from build123d import *

# Parameters (mm, degrees)
PAD005_DEPTH        = 16
FILLET004_R         = 2.5
HOLE005_D           = 4.5
HOLE005_CBORE_D     = 5.6
HOLE005_CBORE_DEPTH = 4.4
SKETCH025_R         = 8.6
PAD007_DEPTH        = 8
PAD008_DEPTH        = 8


with BuildPart() as part:
    # Sketch021 → Pad005 (new body)
    with BuildSketch(Plane.XY):
        with BuildLine():
            Line((-4.795832, 11), (-21, 11))
            Line((-21, 11), (-21, 8))
            Line((-21, 8), (-4.123106, 8))
            ThreePointArc((-4.123106, -8), (9, 0), (-4.123106, 8))
            Line((-21, -8), (-4.123106, -8))
            Line((-21, -12), (-21, -8))
            Line((0, -12), (-21, -12))
            ThreePointArc((0, -12), (11.74734, 2.44949), (-4.795832, 11))
        make_face()
    extrude(amount=PAD005_DEPTH)

    # Fillet004
    fillet004_edges = [part.edges().sort_by_distance(p)[0] for p in [
        (-21, 9.5, 0),
        (-21, 9.5, 16),
        (-21, -10, 16),
        (-21, -10, 0),
    ]]
    fillet(fillet004_edges, radius=FILLET004_R)

    # Hole005 (through all)
    with Locations(Plane.XZ.offset(12)):
        with Locations((-13, 8)):
            CounterBoreHole(HOLE005_D / 2, HOLE005_CBORE_D / 2, HOLE005_CBORE_DEPTH)

    # Sketch025 → Pad007 (join)
    with BuildSketch(Plane.XY):
        with BuildLine():
            ThreePointArc((18.8, 19.2), (13.143146, 16.856854), (10.8, 11.2))
            Line((10.8, -11.2), (10.8, 11.2))
            ThreePointArc((10.8, -11.2), (13.143146, -16.856854), (18.8, -19.2))
            Line((55.2, -19.2), (18.8, -19.2))
            ThreePointArc((55.2, -19.2), (60.856854, -16.856854), (63.2, -11.2))
            Line((63.2, 11.2), (63.2, -11.2))
            ThreePointArc((63.2, 11.2), (60.856854, 16.856854), (55.2, 19.2))
            Line((18.8, 19.2), (55.2, 19.2))
        make_face()
        with Locations((37, 0)):
            Circle(SKETCH025_R, mode=Mode.SUBTRACT)
        with BuildLine():
            ThreePointArc((18.8, 18), (13.991674, 16.008326), (12, 11.2))
            Line((12, 11.2), (12, 1))
            Line((12, 1), (27.251154, 1))
            ThreePointArc((36.4, 9.781615), (30.213702, 7.070089), (27.251154, 1))
            Line((36.4, 18), (36.4, 9.781615))
            Line((18.8, 18), (36.4, 18))
        make_face(mode=Mode.SUBTRACT)
        with BuildLine():
            ThreePointArc((62, 11.2), (60.008326, 16.008326), (55.2, 18))
            Line((37.6, 18), (55.2, 18))
            Line((37.6, 9.781615), (37.6, 18))
            ThreePointArc((37.6, -9.781615), (46.8, 0), (37.6, 9.781615))
            Line((37.6, -18), (37.6, -9.781615))
            Line((55.2, -18), (37.6, -18))
            ThreePointArc((55.2, -18), (60.008326, -16.008326), (62, -11.2))
            Line((62, 11.2), (62, -11.2))
        make_face(mode=Mode.SUBTRACT)
        with BuildLine():
            ThreePointArc((12, -11.2), (13.991674, -16.008326), (18.8, -18))
            Line((36.4, -18), (18.8, -18))
            Line((36.4, -9.781615), (36.4, -18))
            ThreePointArc((27.251154, -1), (30.213702, -7.070089), (36.4, -9.781615))
            Line((12, -1), (27.251154, -1))
            Line((12, -11.2), (12, -1))
        make_face(mode=Mode.SUBTRACT)
    extrude(amount=PAD007_DEPTH)

    # Sketch026 → Pad008 (join)
    with BuildSketch(Plane.XY):
        with BuildLine():
            ThreePointArc((5.838182, 10.484066), (8.996246, 10.358804), (10.967642, 12.82916))
            Line((10.967642, 12.82916), (10.967642, -12.82916))
            ThreePointArc((10.967642, -12.82916), (8.996246, -10.358804), (5.838182, -10.484066))
            Line((5.838182, -10.484066), (4.427288, -7.950416))
            ThreePointArc((4.427288, -7.950416), (9.1, 0), (4.427288, 7.950416))
            Line((5.838182, 10.484066), (4.427288, 7.950416))
        make_face()
    extrude(amount=PAD008_DEPTH)


solid = part.part
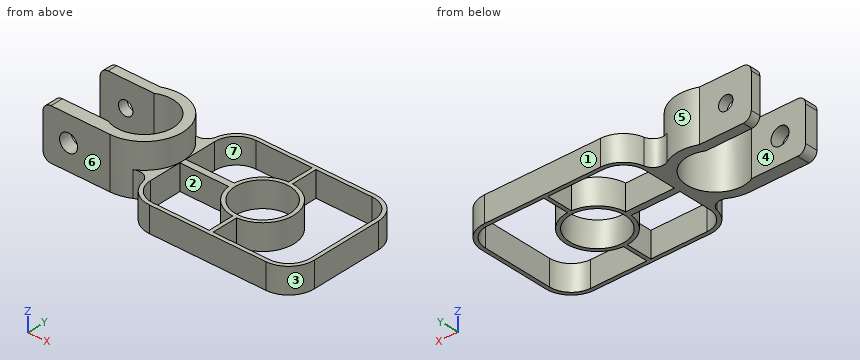
Part model, mm, in its own coordinate system. Face numbers are marked on the shaded views. A direction names the side the tool comes from. Coordinates: 2 decimals unless noted, no trailing zeros. Write each loop counter-clockwise with the first axis right and the second up, starting at its lowest first coordinate (ties: lowest second). Pieces come first, ordered by that corner, then holes. Notation, with made-up numbers: M 41.5,-12.5 L 93.5,-12.5 A18 ccw 93.5,15.5 Z; hole C -27,41.25 d7. An arc over 180 degrees is marked long. Return JSON: item names as keys, results as strings.
1. Saw through at C-C, the plane x = -13. Write the cut outline in (y, z), then the cut area to 3 significant figures.
Determined:
{"outline": "M -12,0 L -8,0 L -8,5.2 L -12,5.2 Z; M -12,10.8 L -8,10.8 L -8,16 L -12,16 Z; M 8,0 L 11,0 L 11,5.75 L 8,5.75 Z; M 8,10.25 L 11,10.25 L 11,16 L 8,16 Z", "area": "76.1 mm²"}
2. Saw through at B-B, the plane y = 0. Write the cut outline in (x, z).
Determined:
{"outline": "M 9,0 L 28.4,0 L 28.4,8 L 12,8 L 12,16 L 9,16 Z; M 45.6,0 L 46.8,0 L 46.8,8 L 45.6,8 Z; M 62,0 L 63.2,0 L 63.2,8 L 62,8 Z"}
3. Pull direction X, two halves, no side cores. Call the marked faces 1, 2 and 3: pulls with the +X half, pulls with the -X half, needs draft (parallel to the pull), parting line crosses it, or undercut.
Determined:
{"face 1": "needs draft", "face 2": "undercut", "face 3": "pulls with the +X half"}
4. Saw through at D-D, the plane z = 14.75. Write the cut outline in (x, y), then the cut area to 3 significant figures.
Determined:
{"outline": "M -20.67,-12 L 0,-12 A12 ccw long -4.8,11 L -20.67,11 L -20.67,8 L -4.12,8 A9 cw long -4.12,-8 L -20.67,-8 Z", "area": "241 mm²"}
5. Probe L1, parallel to Y at x = 18.5, z = 3.75; L2, parallel to Z at x = -13, y = -9; L3, parallel to Y at x = 51, z = 3.5. List the from-to ranges inside material, lowest first.
Determined:
{"L1": "-19.19 to -17.99, -1 to 1, 17.99 to 19.19", "L2": "0 to 5.2, 10.8 to 16", "L3": "-19.2 to -18, 18 to 19.2"}
6. Saw through at A-A, the plane x = 23. Write the cut outline in (y, z).
Determined:
{"outline": "M -19.2,0 L -18,0 L -18,8 L -19.2,8 Z; M -1,0 L 1,0 L 1,8 L -1,8 Z; M 18,0 L 19.2,0 L 19.2,8 L 18,8 Z"}
7. 3-axis set-ups, long thin cutter, end or side, ignore diameter. For the marked faces 4, 5, 6 and 7: which of +Z, -Z, +X, -X, +Y, -Y reach the whole face in a straight line?
Determined:
{"face 4": "+Z, -Z, -X", "face 5": "+Z", "face 6": "+Z, -Z, -X, -Y", "face 7": "+Z, -Z"}
8. Flat gauge pins, fed straight in: pin 1 Ø3.5 at (x, z) = (-13, 8) entering from +Y; pin 2 Ø5 at (x, z) = (-9.5, 10) entering from +Y; pin 3 Ø6.5 at (y, z) = (1.5, 2) entering from -X; pin 4 Ø5 at (x, z) = (-12.5, 5.5) entering from -Y. Where does each tip first touch, or does it go through?
Determined:
{"pin 1": "through", "pin 2": "y = 11", "pin 3": "x = 7.64", "pin 4": "y = -12"}
